Autodesk Inventor part; units mm, degrees
ref_plane "YZ Plane" through (0, 0, 0) normal (1, 0, 0) x (0, 1, 0)
ref_plane "XZ Plane" through (0, 0, 0) normal (0, 1, 0) x (-1, 0, 0)
ref_plane "XY Plane" through (0, 0, 0) normal (0, 0, 1) x (1, 0, 0)
sketch "Sketch1" plane through (0, 0, 0) normal (0, 1, 0) x (-1, 0, 0)
  circle A0 centre (0, 0) radius 4.315
  line L0 (0, 11) -> (0, 22.5) construction
  line L1 (4.315, 11) -> (4.315, 22.5)
  line L2 (-4.315, 22.5) -> (-4.315, 11)
  arc A1 (-4.315, 11) -> (4.315, 11) centre (0, 11) ccw
  arc A2 (4.315, 22.5) -> (-4.315, 22.5) centre (0, 22.5) ccw
  point P0 (0, 16.75)
  dimension "d0" = 8.63
  dimension "d1" = 11.5
  dimension "d2" = 11
extrude "Extrusion1" add sketch "Sketch1" along normal blind 0.5
sketch "Sketch2" plane through (0, 0.5, 0) normal (0, 1, 0) x (1, 0, 0)
  line L0 (-5, -33.5) -> (53.88, -33.5)
  line L1 (61.38, -26) -> (61.38, 114)
  line L2 (53.88, 121.5) -> (-5, 121.5)
  line L3 (-12.5, 114) -> (-12.5, -26)
  circle A0 centre (0, 0) radius 4.315
  line L4 (-4.315, -11) -> (-4.315, -22.5)
  arc A1 (4.315, -11) -> (-4.315, -11) centre (0, -11) ccw
  line L5 (4.315, -22.5) -> (4.315, -11)
  arc A2 (-4.315, -22.5) -> (4.315, -22.5) centre (0, -22.5) ccw
  arc A3 (-12.5, -26) -> (-5, -33.5) centre (-5, -26) ccw
  arc A4 (53.88, -33.5) -> (61.38, -26) centre (53.88, -26) ccw
  arc A5 (61.38, 114) -> (53.88, 121.5) centre (53.88, 114) ccw
  arc A6 (-5, 121.5) -> (-12.5, 114) centre (-5, 114) ccw
  point P0 (61.38, 121.5)
  point P1 (-12.5, 121.5)
  dimension "d5" = 73.88
  dimension "d6" = 155
  dimension "d7" = 33.5
  dimension "d8" = 12.5
  dimension "d9" = 7.5
extrude "Extrusion2" add sketch "Sketch2" along normal blind 8.15 contours A3 L3 A6 L2 A5 L1 A4 L0 | A0 | A1 L5 A2 L4
fillet "Fillet1" radius 4 16 edges at (-10.3033, 0.5, -119.3033) (24.44, 0.5, -121.5) (59.1833, 0.5, -119.3033) (61.38, 0.5, -44) (59.1833, 0.5, 31.3033) (24.44, 0.5, 33.5) (-10.3033, 0.5, 31.3033) (-12.5, 0.5, -44) (-10.3033, 8.65, 31.3033) (24.44, 8.65, 33.5) (59.1833, 8.65, 31.3033) (61.38, 8.65, -44) (59.1833, 8.65, -119.3033) (24.44, 8.65, -121.5) (-10.3033, 8.65, -119.3033) (-12.5, 8.65, -44)
sketch "Sketch3" plane through (-12.5, 4.65, -114) normal (-1, 0, 0) x (0, 0, 1)
  line L0 (0, 0) -> (140, 0)
  line L1 (118.5, 0) -> (98.5, 0) construction
  line L2 (118.5, 1) -> (98.5, 1)
  line L3 (98.5, -1) -> (118.5, -1)
  arc A0 (118.5, -1) -> (118.5, 1) centre (118.5, 0) ccw
  arc A1 (98.5, 1) -> (98.5, -1) centre (98.5, 0) ccw
  line L4 (82, 0) -> (91, 0) construction
  line L5 (82, -1) -> (91, -1)
  line L6 (91, 1) -> (82, 1)
  arc A2 (82, 1) -> (82, -1) centre (82, 0) ccw
  arc A3 (91, -1) -> (91, 1) centre (91, 0) ccw
  line L7 (147.5, -0.15) -> (147.5, 0)
  point P0 (114, -4.65)
  point P1 (108.5, 0)
  point P2 (86.5, 0)
  dimension "d13" = 20
  dimension "d14" = 2
  dimension "d17" = 9
  dimension "d18" = 2
  dimension "d19" = 29
  dimension "d20" = 7.5
extrude "Extrusion3" add sketch "Sketch3" along normal blind 0.75
properties part number "00_Huawei_P20"
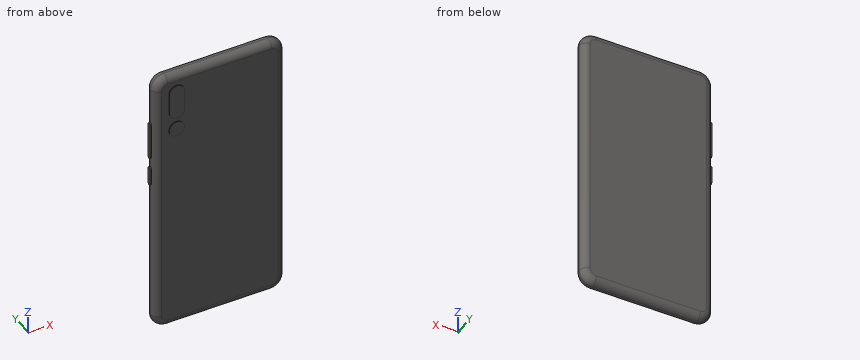
For this review, take the finished solid that the model builds, in its own axes (mm). Round coordinates to 2 decimals unless told otherwise and drop trailing zeros. Loops run counter-clockwise (first coordinate to the right, second up) from the corner with the lowest first, then second, coordinate; pieces in that order, holes last.
Q1. Insertion check: pin 1 Ø4 at (x, z) = (29.5, -96.5) entering from -Y; pin 2 Ø1.1 at (y, z) = (5.5, -29) entering from +X; pin 3 Ø3 at (y, z) = (7.5, -54.5) entering from -X. Each pin has a flat end and moves straight along its axis. Give the tip position at first contact, or say it passes through.
Result sheet:
pin 1: stops at y = 0.5
pin 2: stops at x = 61.37
pin 3: stops at x = -12.27
Q2. Add section D-D on z = -107. Write out the cut boundary in (x, y).
Result sheet:
outline: (-12.5, 4.5) arc R4 ccw to (-8.5, 0.5) - (57.38, 0.5) arc R4 ccw to (61.38, 4.5) - (61.38, 4.65) arc R4 ccw to (57.38, 8.65) - (-8.5, 8.65) arc R4 ccw to (-12.5, 4.65) - close
Q3. To check wall thickness, follow line 1 along Y through (x, z) = (42.5, 16); line 2 along Z through (x, y) = (58, 5.75); line 3 along X through (y, z) = (2.5, 27). State the ranges of each line that lie inside material, in increasing order.
Result sheet:
line 1: y = 0.5 to 8.65
line 2: z = -120.08 to 32.08
line 3: x = -11.89 to 60.77
Q4. Add section B-B on z = 14. Write out the cut boundary in (x, y) (3 decimals), plus the area to 3 significant figures.
Result sheet:
outline: (-12.5, 4.5) arc R4 ccw to (-8.5, 0.5) - (-4.315, 0.5) - (-4.315, 0) - (4.315, 0) - (4.315, 0.5) - (57.38, 0.5) arc R4 ccw to (61.38, 4.5) - (61.38, 4.65) arc R4 ccw to (57.38, 8.65) - (-8.5, 8.65) arc R4 ccw to (-12.5, 4.65) - close
area: 593 mm2
Q5. Add section A-A on x = 46. Write out the cut boundary in (y, z).
Result sheet:
outline: (0.5, -117.5) arc R4 ccw to (4.5, -121.5) - (4.65, -121.5) arc R4 ccw to (8.65, -117.5) - (8.65, 29.5) arc R4 ccw to (4.65, 33.5) - (4.5, 33.5) arc R4 ccw to (0.5, 29.5) - close
Q6. Add section C-C on x = 0. Write out the cut boundary in (y, z) (3 decimals).
Result sheet:
outline: (0, -4.315) - (0.5, -4.315) - (0.5, -117.5) arc R4 ccw to (4.5, -121.5) - (4.65, -121.5) arc R4 ccw to (8.65, -117.5) - (8.65, 29.5) arc R4 ccw to (4.65, 33.5) - (4.5, 33.5) arc R4 ccw to (0.5, 29.5) - (0.5, 26.815) - (0, 26.815) - (0, 6.685) - (0.5, 6.685) - (0.5, 4.315) - (0, 4.315) - close
